from build123d import *

# Parameters (mm, degrees)
SKETCH1_R           = 3.25
BOSS_EXTRUDE1_DEPTH = 5
SKETCH2_W           = 32.64938716
SKETCH2_H           = 32.90693226
BOSS_EXTRUDE2_DEPTH = 5
SKETCH3_R           = 10.567193536
BOSS_EXTRUDE3_DEPTH = 25
SKETCH4_R           = 30
BOSS_EXTRUDE4_DEPTH = 10
FILLET1_R           = 3
FILLET2_R           = 0.56
FILLET3_R           = 3


with BuildPart() as part:
    # Sketch1 → Boss-Extrude1 (new body)
    with BuildSketch(Plane(origin=(0, 0, 0), x_dir=(1, 0, 0), z_dir=(0, 1, 0))):
        with BuildLine():
            Line((-24, -4.668943148), (-24, -24))
            Line((-24, -24), (-4.802343178, -24))
            ThreePointArc((-4.802343178, -24), (0, -26.25), (4.802343178, -24))
            Line((4.802343178, -24), (24, -24))
            Line((24, -24), (24, -4.802343178))
            ThreePointArc((24, -4.802343178), (26.25, 0), (24, 4.802343178))
            Line((24, 4.802343178), (24, 24))
            Line((24, 24), (4.802343178, 24))
            ThreePointArc((4.802343178, 24), (0, 26.25), (-4.802343178, 24))
            Line((-4.802343178, 24), (-24, 24))
            Line((-24, 24), (-24, 5.04363247))
            ThreePointArc((-24, 5.04363247), (-26.315667945, 0.187344661), (-24, -4.668943148))
        make_face()
        with Locations(Location((-20.065667945, 0.187344661, 0), (0, 0, 270))):
            Circle(SKETCH1_R, mode=Mode.SUBTRACT)
        with Locations(Location((0, 20, 0), (0, 0, 270))):
            Circle(SKETCH1_R, mode=Mode.SUBTRACT)
        with Locations(Location((20, 0, 0), (0, 0, 270))):
            Circle(SKETCH1_R, mode=Mode.SUBTRACT)
        with Locations(Location((0, -20, 0), (0, 0, 270))):
            Circle(SKETCH1_R, mode=Mode.SUBTRACT)
        with BuildLine():
            Line((-16, 16), (-4.802343178, 16))
            ThreePointArc((-4.802343178, 16), (0, 13.75), (4.802343178, 16))
            Line((4.802343178, 16), (16, 16))
            Line((16, 16), (16, 4.802343178))
            ThreePointArc((16, 4.802343178), (13.75, 0), (16, -4.802343178))
            Line((16, -4.802343178), (16, -16))
            Line((16, -16), (4.802343178, -16))
            ThreePointArc((4.802343178, -16), (0, -13.75), (-4.802343178, -16))
            Line((-4.802343178, -16), (-16, -16))
            Line((-16, -16), (-16, -4.559532645))
            ThreePointArc((-16, -4.559532645), (-13.815667945, 0.187344661), (-16, 4.934221967))
            Line((-16, 4.934221967), (-16, 16))
        make_face(mode=Mode.SUBTRACT)
    extrude(amount=BOSS_EXTRUDE1_DEPTH)

    # Sketch2 → Boss-Extrude2 (add)
    with BuildSketch(Plane.XZ):
        Rectangle(SKETCH2_W, SKETCH2_H)
    extrude(amount=-BOSS_EXTRUDE2_DEPTH)

    # Sketch3 → Boss-Extrude3 (add)
    with BuildSketch(Plane(origin=(0, 0, 0), x_dir=(-1, 0, 0), z_dir=(0, -1, 0))):
        with Locations(Location((0, 0, 0), (0, 0, 270))):
            Circle(SKETCH3_R)
    extrude(amount=BOSS_EXTRUDE3_DEPTH)

    # Sketch4 → Boss-Extrude4 (add)
    with BuildSketch(Plane(origin=(0, -25, 0), x_dir=(-1, 0, 0), z_dir=(0, -1, 0))):
        with Locations(Location((0, 0, 0), (0, 0, 90))):
            Circle(SKETCH4_R)
    extrude(amount=BOSS_EXTRUDE4_DEPTH)

    # Fillet1
    fillet1_edges = [part.edges().sort_by_distance(p)[0] for p in [
        (0, 0, -10.567193536),
    ]]
    fillet(fillet1_edges, radius=FILLET1_R)

    # Fillet2
    fillet2_edges = [part.edges().sort_by_distance(p)[0] for p in [
        (0, -35, 30),
    ]]
    fillet(fillet2_edges, radius=FILLET2_R)

    # Fillet3
    fillet3_edges = [part.edges().sort_by_distance(p)[0] for p in [
        (0, -25, -10.567193536),
        (0, -25, 30),
    ]]
    fillet(fillet3_edges, radius=FILLET3_R)


solid = part.part
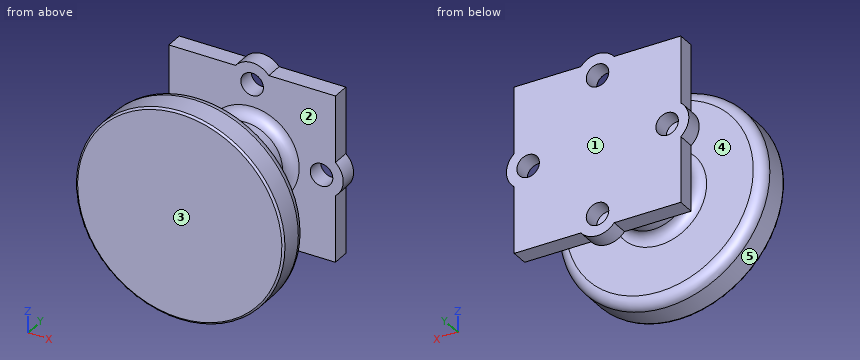
Verification items for the finished model (mm, model axes). Face numbers are marked on the shaded views. A direction names the side the tool comes from. Coordinates: 2 decimals unless noted, no trailing zeros. Write each loop counter-clockwise with the first axis right and the second up, starting at its lowest first coordinate (ties: lowest second). Pieces come first, ordered by that corner, then holes. Notation, with made-up numbers: (40.5, 0) - (57.5, 0) arc R22 cw to (57.5, 34) - close; hole circle Ø7 at (11, 36). An arc over 180 degrees is marked (long way). Answer as a JSON object with one key per item and string values.
(1) Gauge pin test, flat ends, axial feed: pin 1 Ø4 at (x, y) = (-10.5, 2) entering from +Z; pin 2 Ø4 at (x, z) = (-20.07, -0.19) entering from +Y; pin 3 Ø6 at (x, y) = (4.5, -15) entering from +Z; pin 4 Ø8 at (y, z) = (-17.5, -23.5) entering from -X. Record the tip position at first contact, or that the pin passes through.
Report:
{"pin 1": "z = 24", "pin 2": "y = -25", "pin 3": "z = 10.46", "pin 4": "through"}
(2) Tool access check on the marked faces 4 and 5. Record the directions out of +Z, -Z, +X, -X, +Y, -Y that give a thin tool (end or side, any length) a straight path to the whole face; none if there is none.
Report:
{"face 4": "none", "face 5": "-Y"}
(3) Cross-section at A-A on x = 0. Record the cut outline in (y, z).
Report:
{"outline": "(-35, -29.44) arc R0.56 ccw to (-34.44, -30) - (-28, -30) arc R3 ccw to (-25, -27) - (-25, -13.57) arc R3 cw to (-22, -10.57) - (-3, -10.57) arc R3 cw to (0, -13.57) - (0, -16.75) - (5, -16.75) - (5, 16.75) - (0, 16.75) - (0, 13.57) arc R3 cw to (-3, 10.57) - (-22, 10.57) arc R3 cw to (-25, 13.57) - (-25, 27) arc R3 ccw to (-28, 30) - (-34.44, 30) arc R0.56 ccw to (-35, 29.44) - close; (0, -26.25) - (5, -26.25) - (5, -23.25) - (0, -23.25) - close; (0, 23.25) - (5, 23.25) - (5, 26.25) - (0, 26.25) - close"}
(4) Cross-section at D-D on z = 20. Give the number of separate pieces and of enclosed holes in the cut face, plus the area to 3 significant figures.
Report:
{"separate pieces": "3", "enclosed holes": "0", "area": "649 mm^2"}
(5) Cross-section at B-B on z = 0. Record the cut outline in (x, y).
Report:
{"outline": "(-30, -34.44) arc R0.56 ccw to (-29.44, -35) - (29.44, -35) arc R0.56 ccw to (30, -34.44) - (30, -28) arc R3 ccw to (27, -25) - (13.57, -25) arc R3 cw to (10.57, -22) - (10.57, -3) arc R3 cw to (13.57, 0) - (16.75, 0) - (16.75, 5) - (-16.82, 5) - (-16.82, 0) - (-13.57, 0) arc R3 cw to (-10.57, -3) - (-10.57, -22) arc R3 cw to (-13.57, -25) - (-27, -25) arc R3 ccw to (-30, -28) - close; (-26.31, 0) - (-23.31, 0) - (-23.31, 5) - (-26.31, 5) - close; (23.25, 0) - (26.25, 0) - (26.25, 5) - (23.25, 5) - close"}
(6) Mould release check, pull along Y, two halves, no side actions. Record for the marked faces 1, 2 and 3: pulls with the +Y half, pulls with the -Y half, needs draft (parallel to the pull), parting line crosses it, or undercut.
Report:
{"face 1": "pulls with the +Y half", "face 2": "undercut", "face 3": "pulls with the -Y half"}
(7) Thickness scan on line 1 along Y through (x, z) = (18, -12.5); line 2 along X through (y, z) = (3, 20); line 3 along X through (y, z) = (2, 7). Record the ranges inside material, lowest first.
Report:
{"line 1": "-35 to -25, 0 to 5", "line 2": "-24 to -3.25, 3.25 to 24", "line 3": "-24 to 24"}
(8) Cross-section at C-C on y = -19. Record the cut outline in (x, z), plus the area to 3 significant figures.
Report:
{"outline": "circle Ø21.13 at (0, 0)", "area": "351 mm^2"}
